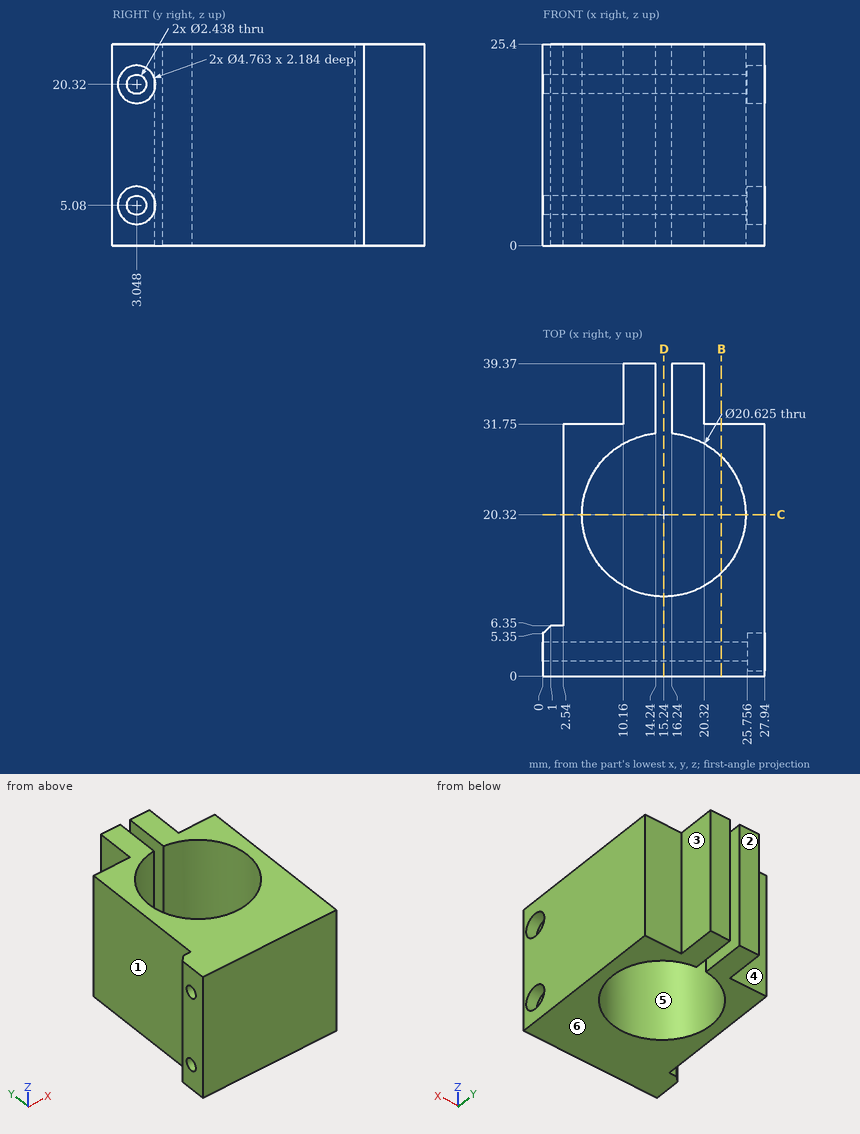
Print and shaded views of the part. All mm, measured from the part's lowest x, y and z. A direction names the side the tool comes from. Round coordinates to 2 decimals unless told otherwise and drop trailing zeros. Write each loop counter-clockwise with the first axis right and the second up, starting at its lowest first coordinate (ties: lowest second). Pieces come first, ordered by that corner, then holes. Notation, with made-up numbers: (-31.5, 87) - (14.5, 87) arc R16 ccw to (14.5, 112) - close; hole circle Ø9 at (4.5, 36). An arc over 180 degrees is marked (long way). Write each question's results on one line, items separated by ' | '. Start each with the question number.
Item 1: Which spindle directions (+Z, -Z, +X, -X, +Y, -Y) get a long thin tool onto all of the face, cutting with end or side? Do the marked faces 1, 2 and 3. Say none if no direction does.
Item 2: Saw through at D-D (x = 15.24). Write the cut outline in (y, z), and give its area (3 significant figures).
Item 3: Saw through at C-C (y = 20.32). Write the cut outline in (x, z).
Item 4: Drop flat-ended pins along their axis: P1, Ø4, axis at x = 23, y = 19, coming from the -Z side; P2, Ø9.5, axis at y = 35.5, z = 12, coming from the -X side; P3, Ø6, axis at x = 23.5, z = 18, coming from the +Y side; P4, Ø4.5, axis at y = 36.5, z = 18, coming from the +X side. Give the stop position or say it passes through.
Item 5: Mould opens along Y. For the marked faces 4, 5 and 6 say: pulls with the +Y half, pulls with the -Y half, needs draft (parallel to the pull), parting line crosses it, or undercut.
Item 6: Saw through at B-B (x = 22.5). Write the cut outline in (y, z).
Item 7: Wall check: L1, parallel to X at y = 20.32, z = 6.5; L2, parallel to Y at x = 26.2, z = 20.32; L3, parallel to Y at x = 26.25, z = 23.25. Give the ranges that are in metal, low to high. Write a range as [from, to].
Results are:
1) face 1: +Z, -Z, -X, +Y | face 2: +Z, -Z, +X, -X, +Y | face 3: +Z, -Z, +X, +Y
2) outline: (0, 0) - (10.01, 0) - (10.01, 25.4) - (0, 25.4) - close; hole circle Ø2.44 at (3.05, 5.08); hole circle Ø2.44 at (3.05, 20.32) | area: 245 mm²
3) outline: (2.54, 0) - (4.93, 0) - (4.93, 25.4) - (2.54, 25.4) - close; (25.55, 0) - (27.94, 0) - (27.94, 25.4) - (25.55, 25.4) - close
4) P1: passes through | P2: stops at x = 2.54 | P3: stops at y = 31.75 | P4: stops at x = 20.32
5) face 4: pulls with the +Y half | face 5: undercut | face 6: needs draft
6) outline: (0, 0) - (13, 0) - (13, 25.4) - (0, 25.4) - close; (27.64, 0) - (31.75, 0) - (31.75, 25.4) - (27.64, 25.4) - close; hole circle Ø2.44 at (3.05, 5.08); hole circle Ø2.44 at (3.05, 20.32)
7) L1: x = [2.54, 4.93], [25.55, 27.94] | L2: y = [0, 0.67], [5.43, 31.75] | L3: y = [0, 31.75]
